```python
from build123d import *

# Parameters (mm, degrees)
F0_R     = 3.5
F2_R     = 5
F4_R     = 2.5
F5_R     = 4
F8_DEPTH = 12.5
F12_R    = 5
F13_R    = 32.75
F9_R     = 4
F11_R    = 31.75


with BuildPart() as f3:
    # F0 (on Top) → F3 section 0
    with BuildSketch(Plane.XY):
        Circle(F0_R)
    # F2 (on offset) → F3 section 1
    with BuildSketch(Plane.XY.offset(27)):
        Circle(F2_R)
    loft()

    # F4 (on Top) → F6 section 0
    with BuildSketch(Plane.XY):
        Circle(F4_R)
    # F5 (on offset) → F6 section 1
    with BuildSketch(Plane.XY.offset(27)):
        Circle(F5_R)
    loft(mode=Mode.SUBTRACT)

    # F7 (on Front) → F8 (cut, symmetric)
    with BuildSketch(Plane.XZ):
        Polygon((12.088457, 9), (-3.5, 0), (12.088457, 0), align=None)
    extrude(amount=F8_DEPTH, both=True, mode=Mode.SUBTRACT)

    # F12 (on offset) → F14 section 0
    with BuildSketch(Plane.XY.offset(27)):
        Circle(F12_R)
    # F13 (on offset) → F14 section 1
    with BuildSketch(Plane.XY.offset(75)):
        Circle(F13_R)
    loft()

    # F9 (on offset) → F15 section 0
    with BuildSketch(Plane.XY.offset(27)):
        Circle(F9_R)
    # F11 (on offset) → F15 section 1
    with BuildSketch(Plane.XY.offset(75)):
        Circle(F11_R)
    loft(mode=Mode.SUBTRACT)


solid = f3.part
```
Model file for the job. Use its own axes, mm. Coordinates: 2 decimals unless noted, no trailing zeros. Order: outer loops, then holes, each group sorted by start corner. A loop starts at its lowest first (then second) coordinate and runs counter-clockwise, first axis right, second up. Notation, with made-up numbers: (86, 0) -> (116, 0) arc R32 ccw to (116, 38) -> close; hole circle Ø3 at (86, -39). An arc over 180 degrees is marked (long way). Answer as a JSON object with one key per item and string values. Group by question number.
1) Cut at A-A, the plane x = 0. Write the cut outline in (y, z).
2) Drill centre lines: L1, parallel to Y at x = 15.5, z = 62; L2, parallel to X at y = -10.5, z = 42; L3, parallel to X at y = -12.5, z = 49. Where is each one in solid material? Low to high.
3) Cut at B-B, the plane z = 25. Write the cut outline in (x, y), then the cut area to 3 significant figures.
4) Flat gauge pins, fed straight in: pin 1 (1.5 mm diameter, centred on y = -24.5, z = 59, fed in from -X); pin 2 (1 mm diameter, centred on x = 16, z = 57.5, fed in from -Y); pin 3 (12 mm diameter, centred on x = 0, z = 22, fed in from +Y); pin 4 (10 mm diameter, centred on y = -2, z = 57.5, fed in from -X). Where does each tip first touch, or does it go through?
5) Cut at C-C, the plane z = 58. Write the cut outline in (x, y), then the cut area to 3 significant figures.
6) Pull direction Y, two halves, no side cores. Call faces 1 (the face through (-3.27, 0.14, 13.89)), 2 (the face through (-3.381, -2.592, 13.689)), 3 (the face through (-1.44, 2.36, 1.19)), 4 (the face through (14.294, 4.501, 46.003)): +Y half, -Y half, draft (parallel to the pull), parting line (faces both ways), or undercut.
Check values:
{
 "1": {"outline": "(-32.75, 75) -> (-5, 27) -> (-3.61, 2.02) -> (-2.61, 2.02) -> (-4, 27) -> (-31.75, 75) -> close; (2.61, 2.02) -> (3.61, 2.02) -> (5, 27) -> (32.75, 75) -> (31.75, 75) -> (4, 27) -> close"},
 "2": {"L1": "y = -19.91 to -18.63, 18.63 to 19.91", "L2": "x = -8.76 to -7.09, 7.09 to 8.76", "L3": "x = -12.56 to -11.1, 11.1 to 12.56"},
 "3": {"outline": "circle Ø9.78 at (0, 0); hole circle Ø7.78 at (0, 0)", "area": "27.6 mm²"},
 "4": {"pin 1": "passes through", "pin 2": "stops at y = -16.64", "pin 3": "stops at y = 5.58", "pin 4": "stops at x = -25.46"},
 "5": {"outline": "circle Ø45.84 at (0, 0); hole circle Ø43.84 at (0, 0)", "area": "141 mm²"},
 "6": {"face 1": "undercut", "face 2": "parting line", "face 3": "draft", "face 4": "undercut"}
}
